from build123d import *

# Parameters (mm, degrees)
FILLET_1_R          = 0.5
SKETCH_2_R          = 1
SKETCH_2_R_2        = 1.25
CUT_EXTRUDE_1_DEPTH = 4
SKETCH_3_R          = 1
SKETCH_3_R_2        = 1.25
CUT_EXTRUDE_2_DEPTH = 4
SKETCH_4_R          = 3.2
CUT_EXTRUDE_3_DEPTH = 1
CUT_EXTRUDE_4_DEPTH = 0.5


with BuildPart() as part:
    # 草图1 → 旋转1 (revolve)
    with BuildSketch(Plane.XY, mode=Mode.PRIVATE) as revolve_1_sk:
        Polygon((2.25, 0), (2.25, 18.5), (4.5, 18.5), (4.5, 18), (6, 18), (6, 15), (16.75, 15), (16.75, 14), (17.3, 14), (17.3, 10.5), (16.75, 10.5), (16.75, 10), (17.3, 10), (17.3, 0), align=None)
    revolve(revolve_1_sk.sketch.rotate(Axis((0, 0, 0), (0, 1, 0)), 90), axis=Axis((0, 0, 0), (0, 1, 0)))

    # 圆角1
    fillet_1_edges = [part.edges().sort_by_distance(p)[0] for p in [
        (0, 0, 17.3),
    ]]
    fillet(fillet_1_edges, radius=FILLET_1_R)

    # 草图2 → 切除-拉伸1 (cut)
    with BuildSketch(Plane(origin=(0, 15, 0), x_dir=(1, 0, 0), z_dir=(0, 1, 0))):
        with Locations(Location((-8, 10.25, 0), (0, 0, 270))):
            Circle(SKETCH_2_R)
        with Locations(Location((8, 10.25, 0), (0, 0, 270))):
            Circle(SKETCH_2_R)
        with Locations(Location((8, -10.25, 0), (0, 0, 270))):
            Circle(SKETCH_2_R)
        with Locations(Location((-8, -10.25, 0), (0, 0, 270))):
            Circle(SKETCH_2_R)
        with Locations(Location((0, 14.75, 0), (0, 0, 270))):
            Circle(SKETCH_2_R_2)
        with Locations(Location((0, -14.75, 0), (0, 0, 90))):
            Circle(SKETCH_2_R_2)
    extrude(amount=-CUT_EXTRUDE_1_DEPTH, mode=Mode.SUBTRACT)

    # 草图3 → 切除-拉伸2 (cut)
    with BuildSketch(Plane.XZ):
        with Locations(Location((0, 6.25, 0), (0, 0, 270))):
            Circle(SKETCH_3_R)
        with Locations(Location((5.25, 5.25, 0), (0, 0, 270))):
            Circle(SKETCH_3_R_2)
        with Locations(Location((6.25, 0, 0), (0, 0, 270))):
            Circle(SKETCH_3_R)
        with Locations(Location((5.25, -5.25, 0), (0, 0, 270))):
            Circle(SKETCH_3_R_2)
        with Locations(Location((0, -6.25, 0), (0, 0, 270))):
            Circle(SKETCH_3_R)
        with Locations(Location((-5.25, -5.25, 0), (0, 0, 270))):
            Circle(SKETCH_3_R_2)
        with Locations(Location((-6.25, 0, 0), (0, 0, 270))):
            Circle(SKETCH_3_R)
        with Locations(Location((-5.25, 5.25, 0), (0, 0, 270))):
            Circle(SKETCH_3_R_2)
    extrude(amount=-CUT_EXTRUDE_2_DEPTH, mode=Mode.SUBTRACT)

    # 草图4 → 切除-拉伸3 (cut)
    with BuildSketch(Plane.XZ):
        with Locations(Location((0, 0, 0), (0, 0, 270))):
            Circle(SKETCH_4_R)
    extrude(amount=-CUT_EXTRUDE_3_DEPTH, mode=Mode.SUBTRACT)

    # 草图5 → 切除-拉伸4 (cut)
    with BuildSketch(Plane(origin=(0, 15, 0), x_dir=(1, 0, 0), z_dir=(0, 1, 0))):
        with BuildLine():
            Line((-13.538235609, -5.613985367), (-9.165063111, -5.613985367))
            ThreePointArc((-9.165063111, -5.613985367), (-8.45795633, -5.321092149), (-8.165063111, -4.613985367))
            Line((-8.165063111, -4.613985367), (-8.165063111, 4.613985367))
            ThreePointArc((-8.165063111, 4.613985367), (-8.45795633, 5.321092149), (-9.165063111, 5.613985367))
            Line((-9.165063111, 5.613985367), (-13.538235609, 5.613985367))
            ThreePointArc((-13.538235609, 5.613985367), (-14.245342391, 5.321092149), (-14.538235609, 4.613985367))
            Line((-14.538235609, 4.613985367), (-14.538235609, -4.613985367))
            ThreePointArc((-14.538235609, -4.613985367), (-14.245342391, -5.321092149), (-13.538235609, -5.613985367))
        make_face()
    extrude(amount=-CUT_EXTRUDE_4_DEPTH, mode=Mode.SUBTRACT)


solid = part.part
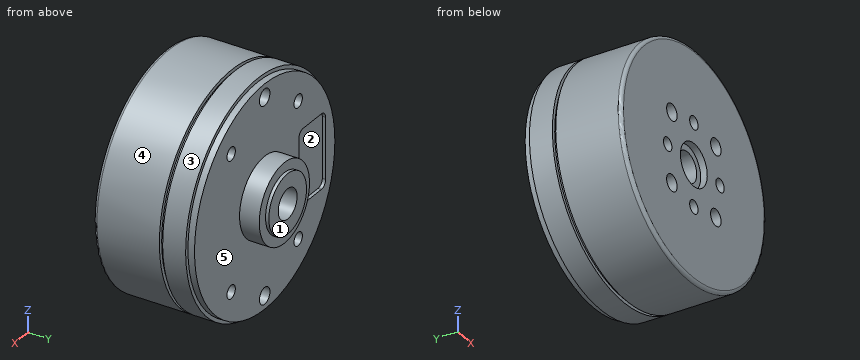
Could you check a few things on this model? Use its own coordinates, in mm. Face numbers are marked on the shaded views. A direction names the side the tool comes from. Give positions to 0.01 mm unless a question says otherwise; leave off trailing zeros. Write each loop counter-clockwise with the first axis right and the second up, starting at its lowest first coordinate (ties: lowest second). Pieces come first, ordered by that corner, then holes. Notation, with made-up numbers: (-21.75, 54) -> (14.25, 54) arc R24 ccw to (14.25, 64) -> close; hole circle Ø6 at (-20, 58.5). An arc over 180 degrees is marked (long way). Answer as a JSON object with one key per item and string values.
Q1. Will these pins go through, and if not, where does the flat tip stop? pin 1 Ø1.2 at (x, z) = (6.25, 0) entering from +Y; pin 2 Ø8 at (x, y) = (-9.5, 3) entering from -Z; pin 3 Ø5 at (x, z) = (-10.5, -1) entering from +Y.
Taken from the geometry:
{"pin 1": "stops at y = 18", "pin 2": "stops at z = -16.4", "pin 3": "stops at y = 15"}
Q2. Please list where these lines run through material, in increasing order: L1, parallel to X at y = 0.7, z = 0; L2, parallel to X at y = 1.4, z = -6.25; L3, parallel to X at y = 9.25, z = 0.
Taken from the geometry:
{"L1": "x = -17.3 to -7.25, -5.25 to -3.2, 3.2 to 5.25, 7.25 to 17.3", "L2": "x = -16.13 to -6, -4.5 to -1, 1 to 4.5, 6 to 16.13", "L3": "x = -17.3 to -2.25, 2.25 to 17.3"}
Q3. Suppose I cut it at A-A on y = 16.5. Write out the boundary of the cut face in (x, z).
Taken from the geometry:
{"outline": "circle Ø12 at (0, 0); hole circle Ø4.5 at (0, 0)"}
Q4. We'd pull the mould along Z, two halves only. Please class the marked faces 1, 2 and 3: released by +Z, released by -Z, zero draft, split by the parting line, or undercut.
Taken from the geometry:
{"face 1": "zero draft", "face 2": "undercut", "face 3": "split by the parting line"}
Q5. Which directions (+Z, -Z, +X, -X, +Y, -Y) give clear straight access to the entire face, cutting with the end or side of a thin tool? Please do the marked faces 4 and 5.
Taken from the geometry:
{"face 4": "+Y, -Y", "face 5": "+Y"}
